Could you check a few things on this drawing? It's one solid part, dimensions in mm from its lowest x, y, z. Round coordinates to 2 decimals unless told otherwise and drop trailing zeros. Answer in a Markdown table with one row per item.
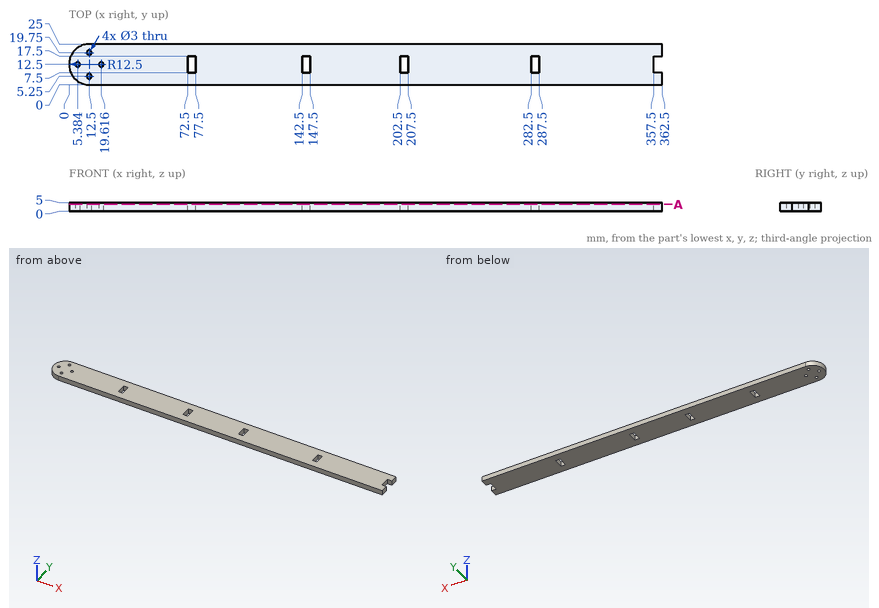
1) I want a section at A-A, the plane z = 4.15. Count the separate pieces of the cut face and the enclosed holes in it, and give its area (3 significant figures).
Response:
| item | result |
|---|---|
| separate pieces | 1 |
| enclosed holes | 8 |
| area | 8,720 mm^2 |
2) For pin 1 (1.5 mm diameter, centred on y = 11, z = 1.5, fed in from -X); pin 2 (3.5 mm diameter, centred on x = 19.62, y = 12.5, fed in from +Z); pin 3 (1 mm diameter, centred on y = 9.5, z = 2, fed in from +X), each with a flat end and sliding along its axis, tell me the tip position at first contact or that it passes through.
Response:
| item | result |
|---|---|
| pin 1 | stops at x = 0.02 |
| pin 2 | stops at z = 5 |
| pin 3 | stops at x = 357.5 |
3) I need wall thicknesses on line 1 (Y direction, x = 12.5, z = 4); line 2 (X direction, y = 17, z = 0.75); line 3 (X direction, y = 16.5, z = 3.85). Which ranges of each line are inside material? Lowest first, please. Write a range as [from, to].
Response:
| item | result |
|---|---|
| line 1 | y = [0, 3.75], [6.75, 18.25], [21.25, 25] |
| line 2 | x = [0.84, 72.5], [77.5, 142.5], [147.5, 202.5], [207.5, 282.5], [287.5, 357.5] |
| line 3 | x = [0.66, 72.5], [77.5, 142.5], [147.5, 202.5], [207.5, 282.5], [287.5, 357.5] |
